from build123d import *

# Parameters (mm, degrees)
F1_DEPTH  = 12
F2_W      = 130
F2_H      = 20
F3_DEPTH  = 5
F4_W      = 105
F4_H      = 20
F5_DEPTH  = 5
F6_R      = 2
F7_DEPTH  = 5
F9_DEPTH  = 5
F10_W     = 135
F10_H     = 20
F10_W_2   = 20
F10_H_2   = 105
F11_DEPTH = 25


with BuildPart() as f1:
    # F0 (on Top) → F1 (new body)
    with BuildSketch(Plane.XY):
        with BuildLine():
            add(Edge.make_bspline(
                [(-116.5, 0), (-116.5, -86.5), (0, -86.5)],
                knots=[3.1415926536, 3.1415926536, 3.1415926536, 4.7123889804, 4.7123889804, 4.7123889804], degree=2, weights=[1, 0.7071067812, 1]))
            Line((-116.5, 0), (-116.5, -86.5))
            Line((-116.5, -86.5), (0, -86.5))
        make_face()
        Polygon((-116.5, -86.5), (-116.5, 0), (-130, 0), (-130, -100), (0, -100), (0, -86.5), align=None)
    extrude(amount=F1_DEPTH)

    # F2 (on face) → F3 (join)
    with BuildSketch(Plane.XZ.offset(100)):
        with Locations((-65, 6)):
            Rectangle(F2_W, F2_H)
    extrude(amount=F3_DEPTH)

    # F4 (on face) → F5 (join)
    with BuildSketch(Plane(origin=(-130, 0, 0), x_dir=(0, -1, 0), z_dir=(-1, 0, 0))):
        with Locations((52.5, 6)):
            Rectangle(F4_W, F4_H)
    extrude(amount=F5_DEPTH)

    # F6 (on face) → F7 (join)
    with BuildSketch(Plane(origin=(0, 0, -4), x_dir=(1, 0, 0), z_dir=(0, 0, -1))):
        Polygon((0, 105), (0, 125), (-155, 125), (-155, 0), (-135, 0), (-135, 105), align=None)
        with Locations((-145, 40)):
            Circle(F6_R, mode=Mode.SUBTRACT)
        with Locations((-145, 85)):
            Circle(F6_R, mode=Mode.SUBTRACT)
        with Locations((-115, 115)):
            Circle(F6_R, mode=Mode.SUBTRACT)
        with Locations((-40, 115)):
            Circle(F6_R, mode=Mode.SUBTRACT)
    extrude(amount=-F7_DEPTH)

    # F8 (on face) → F9 (join)
    with BuildSketch(Plane.XY.offset(16)):
        Polygon((-120, 0), (-135, 0), (-135, -105), (0, -105), (0, -90), (-120, -90), align=None)
    extrude(amount=F9_DEPTH)

    # F10 (on Top) → F11 (cut, symmetric)
    with BuildSketch(Plane.XY):
        with Locations((-87.5, -10)):
            Rectangle(F10_W, F10_H)
        with Locations((-10, -10)):
            Rectangle(F10_W_2, F10_H)
        with Locations((-10, -72.5)):
            Rectangle(F10_W_2, F10_H_2)
    extrude(amount=F11_DEPTH, both=True, mode=Mode.SUBTRACT)


solid = f1.part
Geometry check sheet. Reference: the model listing, model coordinates, mm. A direction names the side the tool comes from. Give positions to 0.01 mm unless a question says otherwise; leave off trailing zeros. Write each loop counter-clockwise with the first axis right and the second up, starting at its lowest first coordinate (ties: lowest second). Pieces come first, ordered by that corner, then holes. Notation, with made-up numbers: (7, 16.25) - (57, 16.25) arc R23 cw to (57, 42.25) - close; hole circle Ø5 at (44.25, 72). An arc over 180 degrees is marked (long way). Put each result on its own line as item: value.
1. Sectioned sample at D-D, the plane z = 18.5. Enter the section's corners in (x, y), plus the area to 4 significant figures.
Ans:
outline: (-135, -105) - (-20, -105) - (-20, -90) - (-120, -90) - (-120, -20) - (-135, -20) - close
area: 2,775 mm²
2. Sectioned sample at C-C, the plane y = -95. Enter the section's corners in (x, z).
Ans:
outline: (-155, -4) - (-130, -4) - (-130, 0) - (-20, 0) - (-20, 12) - (-130, 12) - (-130, 16) - (-20, 16) - (-20, 21) - (-135, 21) - (-135, 1) - (-155, 1) - close
3. Set-up check for faces 5 (the flat face through (-76, -100, -2)), 6 (the flat face through (-135, -62, 11)), 7 (the flat face through (-76, -100, 14)), 8 (the flat face through (-69, -90, 18)): record each of +Z, -Z, +X, -X, +Y, -Y from which the full face is reachable in a straight line by a thin tool's end or side.
Ans:
face 5: -Z, +X, +Y
face 6: +Z, -X, +Y, -Y
face 7: +X, +Y
face 8: +Z, +X, +Y
4. Go/stop test with flat-tipped pins: pin 1 (2.5 mm diameter, centred on y = -44, z = 19.5, fed in from +X); pin 2 (3 mm diameter, centred on y = -67, z = 7.5, fed in from -X); pin 3 (2 mm diameter, centred on x = -76, z = -3, fed in from +Y). Record where each tip stops, or that it passes through.
Ans:
pin 1: stops at x = -120
pin 2: stops at x = -135
pin 3: stops at y = -100
5. Sectioned sample at B-B, the plane x = -115. Enter the section's corners in (y, z), plus the area to 4 significant figures.
Ans:
outline: (-125, -4) - (-117, -4) - (-117, 1) - (-125, 1) - close; (-113, -4) - (-100, -4) - (-100, 0) - (-20, 0) - (-20, 12) - (-100, 12) - (-100, 16) - (-90, 16) - (-90, 21) - (-105, 21) - (-105, 1) - (-113, 1) - close
area: 1,215 mm²
6. Draft check along Z on faces 1 (the flat face through (-130, -59, 14)), 2 (the flat face through (-86, -77, 12)), 3 (the flat face through (-130, -59, -2)), 4 (the flat face through (-118, -108, -4)). Enter one of: +Z half, -Z half, draft (parallel to the pull), parting line (faces both ways), or undercut.
Ans:
face 1: undercut
face 2: undercut
face 3: draft
face 4: -Z half
7. Sectioned sample at A-A, the plane y = -115. Enter the section's corners in (x, z), plus the area to 3 significant figures.
Ans:
outline: (-155, -4) - (-117, -4) - (-117, 1) - (-155, 1) - close; (-113, -4) - (-42, -4) - (-42, 1) - (-113, 1) - close; (-38, -4) - (-20, -4) - (-20, 1) - (-38, 1) - close
area: 635 mm²
8. Thickness scan on line 1 (Y direction, x = -145, z = -2.75); line 2 (X direction, y = -115, z = -0.3); line 3 (X direction, y = -40, z = -1.1). Record the ranges inside material, lowest first.
Ans:
line 1: y = -125 to -87, -83 to -42, -38 to -20
line 2: x = -155 to -117, -113 to -42, -38 to -20
line 3: x = -155 to -147, -143 to -130
